Geometry check sheet. Reference: the model listing, model coordinates, mm. Face numbers are marked on the shaded views. A direction names the side the tool comes from. Round coordinates to 2 decimals unless told otherwise and drop trailing zeros. Loops run counter-clockwise (first coordinate to the right, second up) from the corner with the lowest first, then second, coordinate; pieces in that order, holes last. Notation, with made-up numbers: (-3, -21.5) - (48, -21.5) arc R12 ccw to (48, -10.5) - close; hole circle Ø4 at (88.25, 45). An arc over 180 degrees is marked (long way). Answer as CSV lines item,"result". Start each with the question number.
1) Cross-section at C-C on y = 23.5. Record the boundary of the cut face in (x, z) (3 decimals).
2) Access from +Z, -Z, +X, -X, +Y, -Y to the whole of each face (thin tool, end or side, straight path). Record for the marked faces 4, 5 and 6.
3) Cross-section at B-B on x = -7. Record the boundary of the cut face in (y, z) (3 decimals).
4) Thickness scan on line 1 along X through (y, z) = (1.7, 0) (3 decimals); line 2 along Y through (x, z) = (-2.5, 3.75); line 3 along X through (y, z) = (12.5, -1.5). Record the ranges inside material, lowest first.
5) Cross-section at A-A on y = 17.5. Record the boundary of the cut face in (x, z) (3 decimals).
6) Depth check by flat-ended pin: P1, Ø6, axis at x = 6, y = 8, coming from the -Z side (3 decimals); P2, Ø1.5, axis at x = 9.5, z = 4.5, coming from the +Y side; P3, Ø3, axis at x = 12, z = 1.5, coming from the +Y side. Enter the tip coordinate at first touch or a pass-through.
7) Draft check along Z on the marked faces 1, 2 and 3. Enter one of: released by +Z, released by -Z, zero draft, split by the parting line, or undercut.
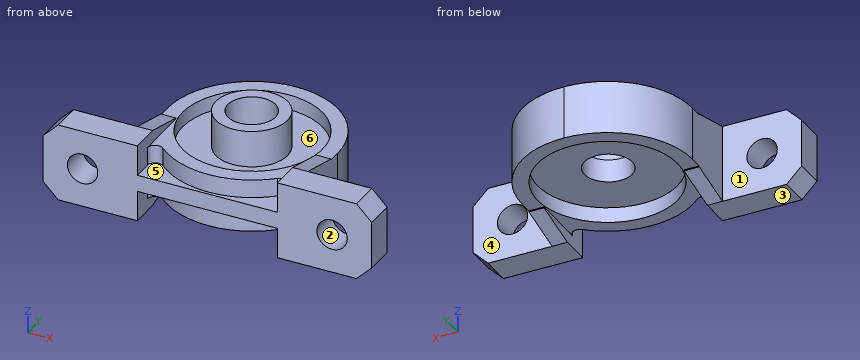
from build123d import *

# Parameters (mm, degrees)
SKETCH1_W                = 55
SKETCH1_H                = 13
BOSS_EXTRUDE1_DEPTH      = 29
CUT_EXTRUDE1_DEPTH       = 14
SKETCH3_OUTSIDE_W        = 69.704
SKETCH3_OUTSIDE_H        = 27.704
SKETCH3_OUTSIDE_W_2      = 28.5
SKETCH3_OUTSIDE_H_2      = 8.89
CUT_EXTRUDE2_DEPTH       = 25
SKETCH5_W                = 2.54
SKETCH5_H                = 7.62
BOSS_EXTRUDE2_DEPTH      = 6.5
BOSS_EXTRUDE2_DEPTH_BACK = 6.5
CHAMFER1_SIZE            = 1.905
CHAMFER1_SIZE2           = 7.62
CHAMFER1_PART_2_SIZE     = 1.905
CHAMFER1_PART_2_SIZE2    = 7.62
CHAMFER2_SIZE            = 7.62
CHAMFER2_SIZE2           = 1.905
CUT_EXTRUDE3_START       = -1.397
CUT_EXTRUDE3_DEPTH       = 6.1030001
CUT_EXTRUDE4_START       = -4.445
SKETCH7_W                = 23.42
SKETCH7_H                = 12.62
CUT_EXTRUDE4_DEPTH       = 3.0550001
SKETCH8_R                = 4
CUT_EXTRUDE5_DEPTH       = 7.5000001
CUT_EXTRUDE5_DEPTH_BACK  = 7.5000001
SKETCH9_R                = 11.71
CUT_EXTRUDE6_DEPTH       = 2.54
CHAMFER3_SIZE            = 2.54
SKETCH10_R               = 2.54
CUT_EXTRUDE7_DEPTH       = 6.0000001
SKETCH11_R               = 6
SKETCH11_R_2             = 4
BOSS_EXTRUDE3_DEPTH      = 6.15


with BuildPart() as part:
    # Sketch1 → Boss-Extrude1 (new body)
    with BuildSketch(Plane(origin=(0, 0, 0), x_dir=(1, 0, 0), z_dir=(0, 1, 0))):
        Rectangle(SKETCH1_W, SKETCH1_H)
    extrude(amount=BOSS_EXTRUDE1_DEPTH)

    # Sketch2 → Cut-Extrude1 (cut, through all)
    with BuildSketch(Plane.XY.offset(6.5)):
        with BuildLine():
            ThreePointArc((-14.25, 14.75), (-10.076271632, 24.826271632), (0, 29))
            Line((0, 29), (-27.5, 29))
            Line((-27.5, 29), (-27.5, 5))
            Line((-27.5, 5), (-14.25, 5))
            Line((-14.25, 5), (-14.25, 14.75))
        make_face()
        with BuildLine():
            Line((14.25, 5), (27.5, 5))
            Line((27.5, 5), (27.5, 29))
            Line((27.5, 29), (0, 29))
            ThreePointArc((0, 29), (10.076271632, 24.826271632), (14.25, 14.75))
            Line((14.25, 14.75), (14.25, 5))
        make_face()
    extrude(amount=-CUT_EXTRUDE1_DEPTH, mode=Mode.SUBTRACT)

    # Sketch3 outside → Cut-Extrude2 (cut, through all)
    with BuildSketch(Plane(origin=(0, 5, 0), x_dir=(1, 0, 0), z_dir=(0, 1, 0))):
        Rectangle(SKETCH3_OUTSIDE_W, SKETCH3_OUTSIDE_H)
        Rectangle(SKETCH3_OUTSIDE_W_2, SKETCH3_OUTSIDE_H_2, mode=Mode.SUBTRACT)
    extrude(amount=CUT_EXTRUDE2_DEPTH, mode=Mode.SUBTRACT)

    # Sketch5 → Boss-Extrude2 (add, two sides)
    with BuildSketch(Plane.XY) as boss_extrude2_sk:
        with Locations((12.98, 8.81)):
            Rectangle(SKETCH5_W, SKETCH5_H)
        with Locations((-12.98, 8.81)):
            Rectangle(SKETCH5_W, SKETCH5_H)
    extrude(amount=BOSS_EXTRUDE2_DEPTH)
    extrude(boss_extrude2_sk.sketch, amount=-BOSS_EXTRUDE2_DEPTH_BACK)

    # Chamfer1
    chamfer1_edges = [part.edges().sort_by_distance(p)[0] for p in [
        (12.98, 12.62, 6.5),
    ]]
    chamfer1_side = [part.faces().sort_by_distance(p)[0] for p in [
        (12.98, 12.62, 5.4725),
    ]]
    chamfer(chamfer1_edges, length=CHAMFER1_SIZE, length2=CHAMFER1_SIZE2, reference=chamfer1_side[0])

    # Chamfer1 part 2
    chamfer1_part_2_edges = [part.edges().sort_by_distance(p)[0] for p in [
        (-12.98, 12.62, 6.5),
    ]]
    chamfer1_part_2_side = [part.faces().sort_by_distance(p)[0] for p in [
        (-12.98, 12.62, 5.4725),
    ]]
    chamfer(chamfer1_part_2_edges, length=CHAMFER1_PART_2_SIZE, length2=CHAMFER1_PART_2_SIZE2, reference=chamfer1_part_2_side[0])

    # Chamfer2
    chamfer2_edges = [part.edges().sort_by_distance(p)[0] for p in [
        (-12.98, 12.62, -6.5),
        (12.98, 12.62, -6.5),
    ]]
    chamfer2_side = [part.faces().sort_by_distance(p)[0] for p in [
        (0, 3.27861046, -6.5),
    ]]
    chamfer(chamfer2_edges, length=CHAMFER2_SIZE, length2=CHAMFER2_SIZE2, reference=chamfer2_side[0])

    # Sketch6 → Cut-Extrude3 (cut, through all)
    with BuildSketch(Plane.XY.offset(CUT_EXTRUDE3_START)):
        with BuildLine():
            Line((11.71, 3.26623755), (11.71, 0))
            Line((11.71, 0), (-11.71, 0))
            Line((-11.71, 0), (-11.71, 3.26623755))
            ThreePointArc((-11.71, 3.26623755), (-10.953777074, 4.427673351), (-9.585695876, 4.205952648))
            ThreePointArc((-9.585695876, 4.205952648), (0, 0.5), (9.585695876, 4.205952648))
            ThreePointArc((9.585695876, 4.205952648), (10.953777074, 4.427673351), (11.71, 3.26623755))
        make_face()
    cut_extrude3 = extrude(amount=-CUT_EXTRUDE3_DEPTH, mode=Mode.SUBTRACT)

    # Sketch7 → Cut-Extrude4 (cut, through all)
    with BuildSketch(Plane.XY.offset(CUT_EXTRUDE4_START)):
        with Locations((0, 6.31)):
            Rectangle(SKETCH7_W, SKETCH7_H)
    cut_extrude4 = extrude(amount=-CUT_EXTRUDE4_DEPTH, mode=Mode.SUBTRACT)

    # Sketch8 → Cut-Extrude5 (cut, two sides)
    with BuildSketch(Plane.XY) as cut_extrude5_sk:
        with Locations((0, 14.5)):
            Circle(SKETCH8_R)
    extrude(amount=CUT_EXTRUDE5_DEPTH, mode=Mode.SUBTRACT)
    extrude(cut_extrude5_sk.sketch, amount=-CUT_EXTRUDE5_DEPTH_BACK, mode=Mode.SUBTRACT)

    # Sketch9 → Cut-Extrude6 (cut)
    with BuildSketch(Plane(origin=(0, 0, -4.445), x_dir=(-1, 0, 0), z_dir=(0, 0, -1))):
        with Locations((0, 14.75)):
            Circle(SKETCH9_R)
    cut_extrude6 = extrude(amount=-CUT_EXTRUDE6_DEPTH, mode=Mode.SUBTRACT)

    # Mirror1: Cut-Extrude3, Cut-Extrude4, Cut-Extrude6 across plane
    add(cut_extrude3.mirror(Plane.XY), mode=Mode.SUBTRACT)
    add(cut_extrude4.mirror(Plane.XY), mode=Mode.SUBTRACT)
    add(cut_extrude6.mirror(Plane.XY), mode=Mode.SUBTRACT)

    # Chamfer3
    chamfer3_edges = [part.edges().sort_by_distance(p)[0] for p in [
        (-27.5, 2.5, 6.5),
        (-27.5, 2.5, -6.5),
        (27.5, 2.5, 6.5),
        (27.5, 2.5, -6.5),
    ]]
    chamfer(chamfer3_edges, length=CHAMFER3_SIZE)

    # Sketch10 → Cut-Extrude7 (cut, through all)
    with BuildSketch(Plane(origin=(0, 5, 0), x_dir=(1, 0, 0), z_dir=(0, 1, 0))):
        with Locations((20.875, 0)):
            Circle(SKETCH10_R)
    cut_extrude7 = extrude(amount=-CUT_EXTRUDE7_DEPTH, mode=Mode.SUBTRACT)

    # Mirror2: Cut-Extrude7 across plane
    add(cut_extrude7.mirror(Plane(origin=(0, 0, 0), x_dir=(0, 0, 1), z_dir=(1, 0, 0))), mode=Mode.SUBTRACT)

    # Sketch11 → Boss-Extrude3 (add)
    with BuildSketch(Plane.XY.offset(1.905)):
        with Locations((0, 14.5)):
            Circle(SKETCH11_R)
        with Locations((0, 14.5)):
            Circle(SKETCH11_R_2, mode=Mode.SUBTRACT)
    extrude(amount=BOSS_EXTRUDE3_DEPTH)


solid = part.part
Answer block:
1,outline,"(-11.247, -4.445) - (-7.782, -4.445) - (-7.782, -1.905) - (7.782, -1.905) - (7.782, -4.445) - (11.247, -4.445) - (11.247, 4.445) - (7.782, 4.445) - (7.782, 1.905) - (-7.782, 1.905) - (-7.782, 4.445) - (-11.247, 4.445) - close"
2,face 4,"+Z, -Z, +X, +Y"
2,face 5,"+Z, -Y"
2,face 6,"+Z"
3,outline,"(0, -1.397) - (2.338, -1.397) - (2.338, -4.445) - (5.363, -4.445) - (5.363, -1.905) - (24.137, -1.905) - (24.137, -4.445) - (27.162, -4.445) - (27.162, 4.445) - (24.137, 4.445) - (24.137, 1.905) - (5.363, 1.905) - (5.363, 4.445) - (2.338, 4.445) - (2.338, 1.397) - (0, 1.397) - close"
4,line 1,"x = -27.5 to -23.415, -18.335 to 18.335, 23.415 to 27.5"
4,line 2,"y = 0.72 to 3.31, 9.05 to 11.38, 17.62 to 19.95, 26.19 to 28.78"
4,line 3,"x = -14.25 to -3.46, 3.46 to 14.25"
5,outline,"(-13.982, -4.445) - (-11.383, -4.445) - (-11.383, -1.905) - (-2.646, -1.905) - (-2.646, 8.055) - (-5.196, 8.055) - (-5.196, 1.905) - (-11.383, 1.905) - (-11.383, 4.445) - (-13.982, 4.445) - close; (2.646, -1.905) - (11.383, -1.905) - (11.383, -4.445) - (13.982, -4.445) - (13.982, 4.445) - (11.383, 4.445) - (11.383, 1.905) - (5.196, 1.905) - (5.196, 8.055) - (2.646, 8.055) - close"
6,P1,"stops at z = -4.445"
6,P2,"stops at y = 26"
6,P3,"stops at y = 24.38"
7,face 1,"zero draft"
7,face 2,"undercut"
7,face 3,"released by -Z"
